Autodesk Inventor part; units mm, degrees
ref_plane "YZ Plane" through (0, 0, 0) normal (1, 0, 0) x (0, 1, 0)
ref_plane "XZ Plane" through (0, 0, 0) normal (0, 1, 0) x (-1, 0, 0)
ref_plane "XY Plane" through (0, 0, 0) normal (0, 0, 1) x (1, 0, 0)
ref_plane "РабПлоскость1" through (0, 0, 0) normal (0, 0, 1) x (1, 0, 0)
sketch "Эскиз1" plane through (0, 0, 0) normal (0, 0, 1) x (1, 0, 0)
  circle A0 centre (7.416, 59.491) radius 2
  circle A1 centre (7.416, 35.509) radius 2
  circle A2 centre (-7.416, 35.509) radius 2
  circle A3 centre (-7.416, 59.491) radius 2
  line L0 (11, 64.0958) -> (-11, 64.0958)
  line L1 (-11, 64.0958) -> (-11, 30.9042)
  line L2 (-11, 30.9042) -> (11, 30.9042)
  line L3 (11, 30.9042) -> (11, 64.0958)
  line L4 (11, 64.0958) -> (-11, 30.9042) construction
  line L5 (7.416, 59.491) -> (-7.416, 35.509) construction
  arc A4 (-24.6917, 37.0776) -> (24.6917, 37.0776) centre (0, 73.5704) ccw
  point P0 (0, 0)
  point P1 (0, 47.5)
  dimension "d0" = 22
extrude "Выдавливание1" add sketch "Эскиз1" along normal blind 11.85 contours L3 L2 L1 L0
fillet "Сопряжение1" radius 3.5 4 edges at (-11, 30.9042, 5.925) (11, 30.9042, 5.925) (11, 64.0958, 5.925) (-11, 64.0958, 5.925)
properties part number "Подставка под солноид"
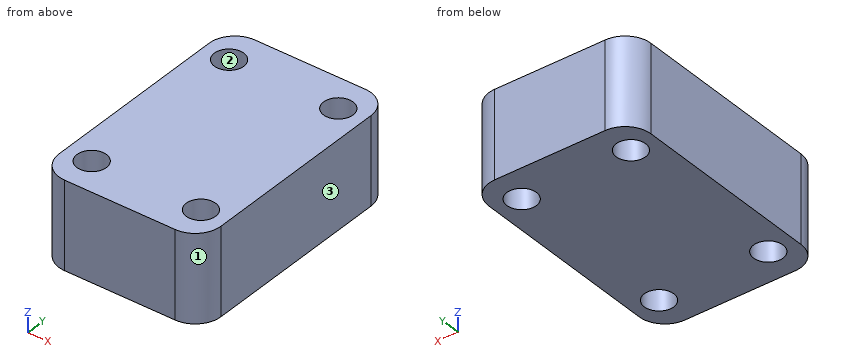
Verification items for the finished model (mm, model axes). Face numbers are marked on the shaded views. Give positions to 0.01 mm unless a question says otherwise; leave off trailing zeros. Order: outer loops, then holes, each group sorted by start corner. A loop starts at its lowest first (then second) coordinate and runs counter-clockwise, first axis right, second up. Notation, with made-up numbers: (2, 86) -> (11, 86) arc R9 cw to (11, 94) -> close; hole circle Ø8 at (4.25, 21). An arc over 180 degrees is marked (long way). One line per item, written item: value.
(1) Sectioned sample at C-C on z = 8.75. Record the cut outline in (x, y), then the cut area to 3 significant figures.
Final values:
outline: (-11, 34.4) arc R3.5 ccw to (-7.5, 30.9) -> (7.5, 30.9) arc R3.5 ccw to (11, 34.4) -> (11, 60.6) arc R3.5 ccw to (7.5, 64.1) -> (-7.5, 64.1) arc R3.5 ccw to (-11, 60.6) -> close; hole circle Ø4 at (-7.42, 35.51); hole circle Ø4 at (-7.42, 59.49); hole circle Ø4 at (7.42, 35.51); hole circle Ø4 at (7.42, 59.49)
area: 669 mm^2
(2) Draft check along Y on the marked faces 1, 2 and 3. Enter one of: pulls with the +Y half, pulls with the -Y half, needs draft (parallel to the pull), parting line crosses it, or undercut.
Final values:
face 1: pulls with the -Y half
face 2: undercut
face 3: needs draft
(3) Sectioned sample at A-A on x = 8.5. Record the cut outline in (y, z).
Final values:
outline: (31.05, 0) -> (33.83, 0) -> (33.83, 11.85) -> (31.05, 11.85) -> close; (37.19, 0) -> (57.81, 0) -> (57.81, 11.85) -> (37.19, 11.85) -> close; (61.17, 0) -> (63.95, 0) -> (63.95, 11.85) -> (61.17, 11.85) -> close
(4) Scan lines: line 1 along Y through (x, z) = (7.25, 7.5); line 2 along Y through (x, z) = (7, 1.5); line 3 along Y through (x, z) = (9.5, 1). Record each from-to range of solid material in increasing order. Write a range as [from, to].
Final values:
line 1: [30.9, 33.52], [37.5, 57.5], [61.48, 64.1]
line 2: [30.9, 33.55], [37.47, 57.53], [61.45, 64.1]
line 3: [31.53, 63.47]
(5) Sectioned sample at B-B on y = 61. Record the cut outline in (x, z).
Final values:
outline: (-10.98, 0) -> (-8.73, 0) -> (-8.73, 11.85) -> (-10.98, 11.85) -> close; (-6.1, 0) -> (6.1, 0) -> (6.1, 11.85) -> (-6.1, 11.85) -> close; (8.73, 0) -> (10.98, 0) -> (10.98, 11.85) -> (8.73, 11.85) -> close
(6) Gauge pin test, flat end, axial feed: pin 1 (3.5 mm diameter, centred on x = 7.416, y = 35.509, fed in from +Z). Record the tip position at first contact, or that the pin passes through.
Final values:
pin 1: through
